Geometry check sheet. Reference: the model listing, model coordinates, mm. Coordinates: 2 decimals unless noted, no trailing zeros. Write each loop counter-clockwise with the first axis right and the second up, starting at its lowest first coordinate (ties: lowest second). Pieces come first, ordered by that corner, then holes. Notation, with made-up numbers: M 52.25,30 L 91.25,30 A11 cw 91.25,48 Z; hole C 78.25,50.5 d7. An arc over 180 degrees is marked long. Write each question's results on one line, items separated by ' | '.
Autodesk Inventor part; units mm, degrees
ref_plane "YZ Plane" through (0, 0, 0) normal (1, 0, 0) x (0, 1, 0)
ref_plane "XZ Plane" through (0, 0, 0) normal (0, 1, 0) x (-1, 0, 0)
ref_plane "XY Plane" through (0, 0, 0) normal (0, 0, 1) x (1, 0, 0)
sketch "草图1" plane through (0, 0, 0) normal (0, 1, 0) x (-1, 0, 0)
  circle A0 centre (0, 0) radius 2
  line L0 (4, 0) -> (2, -3.4641)
  line L1 (2, -3.4641) -> (-2, -3.4641)
  line L2 (-2, -3.4641) -> (-4, 0)
  line L3 (-4, 0) -> (-2, 3.4641)
  line L4 (-2, 3.4641) -> (2, 3.4641)
  line L5 (2, 3.4641) -> (4, 0)
  dimension "d0" = 4
extrude "拉伸2" add sketch "草图1" along normal blind 1.5
thread "螺纹2"
properties part number "螺母"
Q1. Mould release check, pull along X, two halves, no side actions. Record for faces 1 (the cylindrical face through (0, 1, 2)), 2 (the flat face through (0, 1, -3.464)), 3 (the flat face through (3.014, 0.74, 1.708)): pulls with the +X half, pulls with the -X half, needs draft (parallel to the pull), parting line crosses it, or undercut.
Geometry check:
face 1: undercut | face 2: needs draft | face 3: pulls with the +X half
Q2. Sectioned sample at C-C on z = -1.25. Record the cut outline in (x, y).
Geometry check:
outline: M -3.28,0 L -1.56,0 L -1.56,1.5 L -3.28,1.5 Z; M 1.56,0 L 3.28,0 L 3.28,1.5 L 1.56,1.5 Z
Q3. Sectioned sample at A-A on y = 0.9. Record the cut outline in (x, z), and give its area (3 significant figures).
Geometry check:
outline: M -4,0 L -2,-3.46 L 2,-3.46 L 4,0 L 2,3.46 L -2,3.46 Z; hole C 0,0 d4 | area: 29.0 mm2
Q4. Sectioned sample at D-D on x = 3.25. Record the cut outline in (y, z).
Geometry check:
outline: M 0,-1.3 L 1.5,-1.3 L 1.5,1.3 L 0,1.3 Z
Q5. Sectioned sample at B-B on x = 0.75. Record the cut outline in (y, z), and give its area (3 significant figures).
Geometry check:
outline: M 0,-3.46 L 1.5,-3.46 L 1.5,-1.85 L 0,-1.85 Z; M 0,1.85 L 1.5,1.85 L 1.5,3.46 L 0,3.46 Z | area: 4.83 mm2
Q6. Scan lines: probe 1 along Z at (x, y) = (0, 0.7); probe 2 along X at (y, z) = (0.4, 1.5); probe 3 along Z at (x, y) = (1.5, 0.6). Record each from-to range of solid material in increasing order.
Geometry check:
probe 1: z = -3.46 to -2, 2 to 3.46 | probe 2: x = -3.13 to -1.32, 1.32 to 3.13 | probe 3: z = -3.46 to -1.32, 1.32 to 3.46
